Work out the finished part from the listing and answer in its coordinate system (mm). Face numbers are marked on the shaded views. A direction names the side the tool comes from. Give positions to 0.01 mm unless a question says otherwise; leave off trailing zeros. Write each loop counter-clockwise with the first axis right and the second up, starting at its lowest first coordinate (ties: lowest second). Pieces come first, ordered by that corner, then holes.
1) Given pin 1 Ø1.9 at (x, z) = (-28.5, 6) entering from +Y; pin 2 Ø3 at (y, z) = (5, 12) entering from +X; pin 3 Ø1.5 at (y, z) = (5.5, 4.5) entering from +X, each flat-ended and moving along its own axis, determine where each tip first touches the part or whether it passes through.
2) Straight lines are drawn through the part: probe 1 along X at (y, z) = (1.25, 11.25); probe 2 along X at (y, z) = (1.75, 5.25); probe 3 along Y at (x, z) = (26, 8.75). For each, find the intervals that lie inside material, in ascending order.
3) Find section D-D (x = -27). Determine the outline of the cut face in (y, z), plus the area to 3 significant figures.
4) Find section A-A (y = 8.5). Determine the outline of the cut face in (x, z), plus the area to 3 significant figures.
5) A tool of negligible diameter and unlimited length cuts with its end or side. For the marked faces 4 and 5, from which of +Z, -Z, +X, -X, +Y, -Y can it reach the whole face along a straight path? Write none if from no direction.
6) Determine the mould class of the marked faces 1, 2 and 3 for opening direction X: pulls with the +X half, pulls with the -X half, needs draft (parallel to the pull), parting line crosses it, or undercut.
7) Find section C-C (y = 3.25). Determine the outline of the cut face in (x, z).
8) Find section B-B (z = 13.25). Determine the outline of the cut face in (x, y).
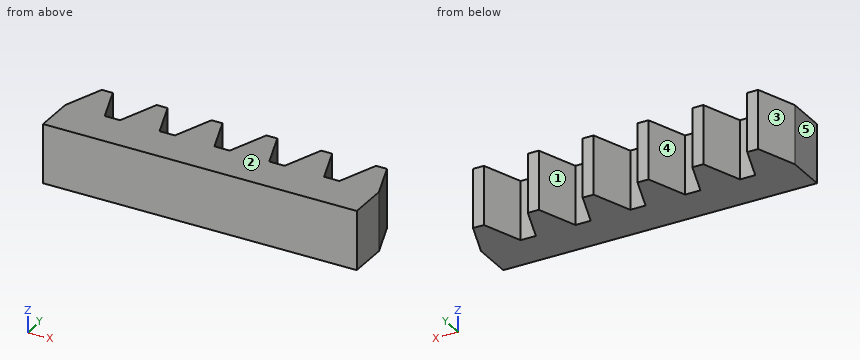
```python
from build123d import *

# Parameters (mm, degrees)
F1_DEPTH = 15


with BuildPart() as f1:
    # F0 (on Top) → F1 (new body)
    with BuildSketch(Plane.XY):
        Polygon((5.589702, 10.04253), (1.95, 0.04253), (-1.948, 0.04253), (-5.587702, 10.04253), (-8.372702, 10.04253), (-12.012405, 0.04253), (-15.910405, 0.04253), (-19.550107, 10.04253), (-22.335107, 10.04253), (-25.974809, 0.04253), (-29.872809, 0.04253), (-33.512512, 10.04253), (-36.297512, 10.04253), (-39.937214, 0.04253), (-39.937214, -9.898053), (39.939214, -9.898053), (39.939214, 0.04253), (36.299512, 10.04253), (33.514512, 10.04253), (29.874809, 0.04253), (25.976809, 0.04253), (22.337107, 10.04253), (19.552107, 10.04253), (15.912405, 0.04253), (12.014405, 0.04253), (8.374702, 10.04253), align=None)
    extrude(amount=F1_DEPTH)


solid = f1.part
```
Results:
1. pin 1: stops at y = 0.04
1. pin 2: stops at x = 38.68
1. pin 3: stops at x = 38.23
2. probe 1: x = -39.5 to -30.31, -25.54 to -16.35, -11.57 to -2.39, 2.39 to 11.57, 16.35 to 25.54, 30.31 to 39.5
2. probe 2: x = -39.32 to -30.49, -25.35 to -16.53, -11.39 to -2.57, 2.57 to 11.39, 16.53 to 25.36, 30.5 to 39.32
2. probe 3: y = -9.9 to 0.04
3. outline: (-9.9, 0) - (0.04, 0) - (0.04, 15) - (-9.9, 15) - close
3. area: 149 mm2
4. outline: (-36.86, 0) - (-32.95, 0) - (-32.95, 15) - (-36.86, 15) - close; (-22.9, 0) - (-18.99, 0) - (-18.99, 15) - (-22.9, 15) - close; (-8.93, 0) - (-5.03, 0) - (-5.03, 15) - (-8.93, 15) - close; (5.03, 0) - (8.94, 0) - (8.94, 15) - (5.03, 15) - close; (18.99, 0) - (22.9, 0) - (22.9, 15) - (18.99, 15) - close; (32.95, 0) - (36.86, 0) - (36.86, 15) - (32.95, 15) - close
4. area: 352 mm2
5. face 4: +Z, -Z, +Y
5. face 5: +Z, -Z, -X, +Y, -Y
6. face 1: undercut
6. face 2: needs draft
6. face 3: pulls with the -X half
7. outline: (-38.77, 0) - (-31.04, 0) - (-31.04, 15) - (-38.77, 15) - close; (-24.81, 0) - (-17.08, 0) - (-17.08, 15) - (-24.81, 15) - close; (-10.84, 0) - (-3.12, 0) - (-3.12, 15) - (-10.84, 15) - close; (3.12, 0) - (10.85, 0) - (10.85, 15) - (3.12, 15) - close; (17.08, 0) - (24.81, 0) - (24.81, 15) - (17.08, 15) - close; (31.04, 0) - (38.77, 0) - (38.77, 15) - (31.04, 15) - close
8. outline: (-39.94, -9.9) - (39.94, -9.9) - (39.94, 0.04) - (36.3, 10.04) - (33.51, 10.04) - (29.87, 0.04) - (25.98, 0.04) - (22.34, 10.04) - (19.55, 10.04) - (15.91, 0.04) - (12.01, 0.04) - (8.37, 10.04) - (5.59, 10.04) - (1.95, 0.04) - (-1.95, 0.04) - (-5.59, 10.04) - (-8.37, 10.04) - (-12.01, 0.04) - (-15.91, 0.04) - (-19.55, 10.04) - (-22.34, 10.04) - (-25.97, 0.04) - (-29.87, 0.04) - (-33.51, 10.04) - (-36.3, 10.04) - (-39.94, 0.04) - close
